```python
from build123d import *

# Parameters (mm, degrees)
EXTRUDE1_START = -7.2009
SKETCH1_R      = 15.08125
SKETCH1_R_2    = 7.95
EXTRUDE1_DEPTH = 14.4018
CHAMFER1_SIZE  = 1


with BuildPart() as part:
    # Sketch1 → Extrude1 (new body)
    with BuildSketch(Plane.XY.offset(EXTRUDE1_START)):
        Circle(SKETCH1_R)
        Circle(SKETCH1_R_2, mode=Mode.SUBTRACT)
    extrude(amount=EXTRUDE1_DEPTH)

    # Chamfer1
    chamfer1_edges = [part.edges().sort_by_distance(p)[0] for p in [
        (-15.08125, 0, -7.2009),
        (-15.08125, 0, 7.2009),
    ]]
    chamfer(chamfer1_edges, length=CHAMFER1_SIZE)

    # Sketch2 → Revolve1 (revolve)
    with BuildSketch(Plane(origin=(0, 0, 0), x_dir=(0, 0, -1), z_dir=(1, 0, 0))):
        with BuildLine():
            Line((7.95, 7.94), (-7.95, 7.94))
            Line((-7.95, 7.94), (-7.95, 10.895295258))
            ThreePointArc((-7.95, 10.895295258), (0, 13.4874), (7.95, 10.895295258))
            Line((7.95, 10.895295258), (7.95, 7.94))
        make_face()
    revolve(axis=Axis((0, 0, -11.466432169), (0, 0, 1)))

    # Sketch2_2 → Cut-Revolve1 (revolve, cut)
    with BuildSketch(Plane(origin=(0, 0, 0), x_dir=(0, 0, -1), z_dir=(1, 0, 0))):
        with BuildLine():
            Line((7.95, 7.94), (-7.95, 7.94))
            Line((-7.95, 7.94), (-7.95, 10.895295258))
            ThreePointArc((-7.95, 10.895295258), (0, 13.4874), (7.95, 10.895295258))
            Line((7.95, 10.895295258), (7.95, 7.94))
        make_face()
    revolve(axis=Axis((0, 0, -11.466432169), (0, 0, 1)), mode=Mode.SUBTRACT)


solid = part.part
```
Geometry check sheet. Reference: the model listing, model coordinates, mm. Coordinates: 2 decimals unless noted, no trailing zeros. Order: outer loops, then holes, each group sorted by start corner. A loop starts at its lowest first (then second) coordinate and runs counter-clockwise, first axis right, second up. Notation, with made-up numbers: (22.5, -19.5) - (66.5, -19.5) arc R13 ccw to (66.5, 2.5) - close; hole circle Ø3 at (72, 12). An arc over 180 degrees is marked (long way). Answer in a Markdown table with one row per item. Add a question column.
1. Section check A-A (x = 0). Enter the section's corners in (y, z).
2. Material ranges on L1, parallel to Y at x = 9, z = -3.5; L2, parallel to Y at x = 0, z = -5.5; L3, parallel to X at y = -1, z = -1, recorded low to high. Write a range as [from, to].
3. Section check D-D (z = 3.5). Enter the section's corners in (x, y), plus the area to 3 significant figures.
4. Section check C-C (z = -1.75). Enter the section's corners in (x, y).
5. Gauge pin test, flat ends, axial feed: pin 1 Ø1.5 at (y, z) = (9.5, -4) entering from +X; pin 2 Ø5 at (x, z) = (6.5, -1) entering from -Y; pin 3 Ø2 at (x, z) = (-11.5, 4.5) entering from +Y. Record the tip position at first contact, or that the pin passes through.
Data:
| question | item | result |
|---|---|---|
| 1 | outline | (-15.08, -6.2) - (-14.08, -7.2) - (-11.4, -7.2) arc R13.49 cw to (-11.4, 7.2) - (-14.08, 7.2) - (-15.08, 6.2) - close; (11.4, -7.2) - (14.08, -7.2) - (15.08, -6.2) - (15.08, 6.2) - (14.08, 7.2) - (11.4, 7.2) arc R13.49 cw to start |
| 2 | L1 | y = [-12.1, -9.42], [9.42, 12.1] |
| 2 | L2 | y = [-15.08, -12.32], [12.32, 15.08] |
| 2 | L3 | x = [-15.05, -13.41], [13.41, 15.05] |
| 3 | outline | circle Ø30.16 at (0, 0); hole circle Ø26.05 at (0, 0) |
| 3 | area | 182 mm² |
| 4 | outline | circle Ø30.16 at (0, 0); hole circle Ø26.75 at (0, 0) |
| 5 | pin 1 | stops at x = 12.28 |
| 5 | pin 2 | stops at y = -14.54 |
| 5 | pin 3 | stops at y = 10.83 |
